from build123d import *

# Parameters (mm, degrees)
SKETCH_1_W          = 400
SKETCH_1_H          = 60
SKETCH_1_R          = 1.6
SKETCH_1_W_2        = 21
SKETCH_1_H_2        = 21
SKETCH_1_W_3        = 240
SKETCH_1_H_3        = 75
SKETCH_1_R_2        = 20
EXTRUDE_1466_DEPTH  = 3
SKETCH_2_R          = 2.05
SKETCH_2_R_2        = 2.1
CUT_EXTRUDE_1_DEPTH = 250.229009796
FILLET_1_R          = 5
SKETCH1_R           = 2.1
CUT_EXTRUDE4_DEPTH  = 250.229009796


with BuildPart() as part:
    # 草图1 → Extrude 1466 (new body)
    # profile 1 of 2: a face of its own
    with BuildSketch(Plane(origin=(0, 0, 0), x_dir=(1, 0, 0), z_dir=(0, 1, 0))):
        with Locations((32.825924772, 16.128249268)):
            Rectangle(SKETCH_1_W, SKETCH_1_H)
        with Locations(Location((-14.674075228, 36.128249268, 0), (0, 0, 270))):
            Circle(SKETCH_1_R, mode=Mode.SUBTRACT)
        with Locations(Location((-14.674075228, 11.128249268, 0), (0, 0, 270))):
            Circle(SKETCH_1_R, mode=Mode.SUBTRACT)
        with Locations(Location((80.325924772, 11.128249268, 0), (0, 0, 270))):
            Circle(SKETCH_1_R, mode=Mode.SUBTRACT)
        with Locations(Location((80.325924772, 36.128249268, 0), (0, 0, 270))):
            Circle(SKETCH_1_R, mode=Mode.SUBTRACT)
        with Locations((32.825924772, 10.628249268)):
            Rectangle(SKETCH_1_W_2, SKETCH_1_H_2, mode=Mode.SUBTRACT)
    # profile 2 of 2: a face of its own
    with BuildSketch(Plane(origin=(0, 0, 0), x_dir=(1, 0, 0), z_dir=(0, 1, 0))):
        with Locations((32.825924772, -51.371750732)):
            Rectangle(SKETCH_1_W_3, SKETCH_1_H_3)
        with Locations(Location((7.825924772, -29.871750732, 0), (0, 0, 270))):
            Circle(SKETCH_1_R, mode=Mode.SUBTRACT)
        with Locations(Location((7.825924772, -79.871750732, 0), (0, 0, 270))):
            Circle(SKETCH_1_R, mode=Mode.SUBTRACT)
        with Locations(Location((57.825924772, -79.871750732, 0), (0, 0, 270))):
            Circle(SKETCH_1_R, mode=Mode.SUBTRACT)
        with Locations(Location((57.825924772, -29.871750732, 0), (0, 0, 270))):
            Circle(SKETCH_1_R, mode=Mode.SUBTRACT)
        with Locations(Location((32.825924772, -54.871750732, 0), (0, 0, 270))):
            Circle(SKETCH_1_R_2, mode=Mode.SUBTRACT)
    extrude(amount=EXTRUDE_1466_DEPTH)

    # 草图2 → 切除-拉伸1 (cut, through all)
    with BuildSketch(Plane(origin=(0, 3, 0), x_dir=(1, 0, 0), z_dir=(0, 1, 0))):
        with Locations(Location((-149.174075228, 29.628249268, 0), (0, 0, 270))):
            Circle(SKETCH_2_R)
        with Locations(Location((-149.174075228, 2.628249268, 0), (0, 0, 270))):
            Circle(SKETCH_2_R)
        with Locations(Location((-121.674075228, 29.628249268, 0), (0, 0, 270))):
            Circle(SKETCH_2_R)
        with Locations(Location((-121.674075228, 2.628249268, 0), (0, 0, 90))):
            Circle(SKETCH_2_R)
        with Locations(Location((-51.674075228, 41.128249268, 0), (0, 0, 270))):
            Circle(SKETCH_2_R_2)
        with Locations(Location((-86.674075228, 41.128249268, 0), (0, 0, 270))):
            Circle(SKETCH_2_R_2)
        with Locations(Location((-51.674075228, -8.871750732, 0), (0, 0, 90))):
            Circle(SKETCH_2_R_2)
        with Locations(Location((-86.674075228, -8.871750732, 0), (0, 0, 90))):
            Circle(SKETCH_2_R_2)
        with Locations(Location((-135.424075228, 41.128249268, 0), (0, 0, 270))):
            Circle(SKETCH_2_R_2)
        with Locations(Location((-135.424075228, -8.871750732, 0), (0, 0, 90))):
            Circle(SKETCH_2_R_2)
        with Locations(Location((201.075924772, -8.871750732, 0), (0, 0, 270))):
            Circle(SKETCH_2_R_2)
        with Locations(Location((201.075924772, 41.128249268, 0), (0, 0, 90))):
            Circle(SKETCH_2_R_2)
        with Locations(Location((152.325924772, -8.871750732, 0), (0, 0, 270))):
            Circle(SKETCH_2_R_2)
        with Locations(Location((117.325924772, -8.871750732, 0), (0, 0, 270))):
            Circle(SKETCH_2_R_2)
        with Locations(Location((152.325924772, 41.128249268, 0), (0, 0, 90))):
            Circle(SKETCH_2_R_2)
        with Locations(Location((117.325924772, 41.128249268, 0), (0, 0, 90))):
            Circle(SKETCH_2_R_2)
        with Locations(Location((187.325924772, 2.628249268, 0), (0, 0, 270))):
            Circle(SKETCH_2_R)
        with Locations(Location((187.325924772, 29.628249268, 0), (0, 0, 90))):
            Circle(SKETCH_2_R)
        with Locations(Location((214.825924772, 2.628249268, 0), (0, 0, 90))):
            Circle(SKETCH_2_R)
        with Locations(Location((214.825924772, 29.628249268, 0), (0, 0, 90))):
            Circle(SKETCH_2_R)
    extrude(amount=-CUT_EXTRUDE_1_DEPTH, mode=Mode.SUBTRACT)

    # 圆角1
    fillet_1_edges = [part.edges().sort_by_distance(p)[0] for p in [
        (-167.174075228, 1.5, 13.871750732),
        (-167.174075228, 1.5, -46.128249268),
        (232.825924772, 1.5, -46.128249268),
        (232.825924772, 1.5, 13.871750732),
        (152.825924772, 1.5, 13.871750732),
        (152.825924772, 1.5, 88.871750732),
        (-87.174075228, 1.5, 88.871750732),
        (-87.174075228, 1.5, 13.871750732),
    ]]
    fillet(fillet_1_edges, radius=FILLET_1_R)

    # Sketch1 → Cut-Extrude4 (cut, through all)
    with BuildSketch(Plane(origin=(0, 0, 0), x_dir=(1, 0, 0), z_dir=(0, 1, 0))):
        with Locations(Location((-72.174075228, -33.871750732, 0), (0, 0, 270))):
            Circle(SKETCH1_R)
        with Locations(Location((-72.174075228, -68.871750732, 0), (0, 0, 270))):
            Circle(SKETCH1_R)
        with Locations(Location((137.825924772, -68.871750732, 0), (0, 0, 90))):
            Circle(SKETCH1_R)
        with Locations(Location((137.825924772, -33.871750732, 0), (0, 0, 90))):
            Circle(SKETCH1_R)
        with BuildLine():
            Line((-42.174075228, -68.871750732), (-42.174075228, -33.871750732))
            ThreePointArc((-42.174075228, -33.871750732), (-32.174075228, -23.871750732), (-22.174075228, -33.871750732))
            Line((-22.174075228, -33.871750732), (-22.174075228, -68.871750732))
            ThreePointArc((-22.174075228, -68.871750732), (-32.174075228, -78.871750732), (-42.174075228, -68.871750732))
        make_face()
        with BuildLine():
            Line((107.825924772, -68.871750732), (107.825924772, -33.871750732))
            ThreePointArc((107.825924772, -33.871750732), (97.825924772, -23.871750732), (87.825924772, -33.871750732))
            Line((87.825924772, -33.871750732), (87.825924772, -68.871750732))
            ThreePointArc((87.825924772, -68.871750732), (97.825924772, -78.871750732), (107.825924772, -68.871750732))
        make_face()
    extrude(amount=CUT_EXTRUDE4_DEPTH, mode=Mode.SUBTRACT)


solid = part.part
Source: CAD feature listing. Evaluate the final solid. Frame: model axes, mm. A direction names the side the tool comes from. Coordinates: 2 decimals unless noted, no trailing zeros. Order: outer loops, then holes, each group sorted by start corner. A loop starts at its lowest first (then second) coordinate and runs counter-clockwise, first axis right, second up. Notation, with made-up numbers: M 21,32.5 L 37,32.5 A20 ccw 37,66.5 Z; hole C 25.5,84 d5. An arc over 180 degrees is marked long. Write each question's results on one line, items separated by ' | '. Start each with the question number.
Item 1: Set-up query: faces 1 (the face through (30, 3, 5)), 2 (the face through (98.046, 1.479, 23.874)). Return all of +Z, -Z, +X, -X, +Y, -Y with unobstructed straight access to the full face (end or side cutting, diameter ignored); none if empty.
Item 2: Line query: probe 1 along X at (y, z) = (2, 54); probe 2 along X at (y, z) = (0.2, -8); probe 3 along Z at (x, y) = (-33, 1.1). Output: solid intervals per line, ascending.
Item 3: Cut plane D-D (x = -104). Return loops of the section in (y, z).
Item 4: First-contact query: pin 1 Ø4 at (x, z) = (-86.67, -41.13) entering from -Y; pin 2 Ø0.9 at (y, z) = (2, 52.5) entering from +X. Flat tips, straight axial feed; report the tip coordinate or a pass-through.
Item 5: Draft query along X for faces 3 (the face through (33.71, 1.48, 34.89)), 4 (the face through (30, 0, 5)). Return one class per face: pulls with the +X half, pulls with the -X half, needs draft (parallel to the pull), parting line crosses it, or undercut.
Item 6: Cut plane C-C (y = 0.95). Count the separate pieces of the cut face and the enclosed holes in it, and give its area (3 significant figures).
Item 7: Cut plane A-A (x = 37.5). Return loops of the section in (y, z), and give its area (3 significant figures).
Item 8: Cut plane B-B (z = 42.5). Return loops of the section in (x, y).
Checked values:
1) face 1: +Z, -Z, +X, -X, +Y | face 2: +Y, -Y
2) probe 1: x = -87.17 to -42.17, -22.17 to 12.84, 52.81 to 87.83, 107.83 to 152.83 | probe 2: x = -167.17 to 22.33, 43.33 to 232.83 | probe 3: z = -46.13 to 23.91, 78.84 to 88.87
3) outline: M 0,-46.13 L 3,-46.13 L 3,13.87 L 0,13.87 Z
4) pin 1: passes through | pin 2: stops at x = 152.83
5) face 3: undercut | face 4: needs draft
6) separate pieces: 1 | enclosed holes: 36 | area: 37,900 mm2
7) outline: M 0,-46.13 L 3,-46.13 L 3,-21.13 L 0,-21.13 Z; M 0,-0.13 L 3,-0.13 L 3,35.43 L 0,35.43 Z; M 0,74.32 L 3,74.32 L 3,88.87 L 0,88.87 Z | area: 225 mm2
8) outline: M -87.17,0 L -42.17,0 L -42.17,3 L -87.17,3 Z; M -22.17,0 L 17.11,0 L 17.11,3 L -22.17,3 Z; M 48.54,0 L 87.83,0 L 87.83,3 L 48.54,3 Z; M 107.83,0 L 152.83,0 L 152.83,3 L 107.83,3 Z
